```python
from build123d import *

# Parameters (mm, degrees)
BOSS_EXTRUDE1_DEPTH = 70
CHAMFER1_SIZE       = 7
FILLET1_R           = 2
SKETCH2_R           = 1.75
SKETCH2_R_2         = 20
CUT_EXTRUDE1_DEPTH  = 23
CUT_EXTRUDE2_START  = -4
SKETCH3_R           = 4.75
SKETCH3_R_2         = 1.75
CUT_EXTRUDE2_DEPTH  = 4
SKETCH5_R           = 20
CUT_EXTRUDE3_DEPTH  = 23


with BuildPart() as part:
    # Sketch1 → Boss-Extrude1 (new body)
    with BuildSketch(Plane.XY):
        Polygon((-55, 0), (0, 0), (0, 55), (-8, 55), (-8, 63), (8, 63), (8, -8), (-63, -8), (-63, 8), (-55, 8), align=None)
    extrude(amount=BOSS_EXTRUDE1_DEPTH)

    # Chamfer1
    chamfer1_edges = [part.edges().sort_by_distance(p)[0] for p in [
        (-8, 63, 35),
        (-63, 8, 35),
    ]]
    chamfer(chamfer1_edges, length=CHAMFER1_SIZE)

    # Fillet1
    fillet1_edges = [part.edges().sort_by_distance(p)[0] for p in [
        (8, 63, 35),
        (8, -8, 35),
        (-63, -8, 35),
    ]]
    fillet(fillet1_edges, radius=FILLET1_R)

    # Sketch2 → Cut-Extrude1 (cut)
    with BuildSketch(Plane.XZ.offset(8)):
        with Locations(Location((-40, 62.5, 0), (0, 0, 270))):
            Circle(SKETCH2_R)
        with Locations(Location((-15, 62.5, 0), (0, 0, 270))):
            Circle(SKETCH2_R)
        with Locations(Location((-15, 7.5, 0), (0, 0, 270))):
            Circle(SKETCH2_R)
        with Locations(Location((-40, 7.5, 0), (0, 0, 270))):
            Circle(SKETCH2_R)
        with Locations(Location((-27.5, 35, 0), (0, 0, 270))):
            Circle(SKETCH2_R_2)
    extrude(amount=-CUT_EXTRUDE1_DEPTH, mode=Mode.SUBTRACT)

    # Sketch3 → Cut-Extrude2 (cut)
    # profile 1 of 4: a face of its own
    with BuildSketch(Plane(origin=(0, 0, 0), x_dir=(1, 0, 0), z_dir=(0, 1, 0)).offset(CUT_EXTRUDE2_START)):
        with Locations(Location((-40, -62.5, 0), (0, 0, 270))):
            Circle(SKETCH3_R)
        with Locations(Location((-40, -62.5, 0), (0, 0, 90))):
            Circle(SKETCH3_R_2, mode=Mode.SUBTRACT)
    # profile 2 of 4: a face of its own
    with BuildSketch(Plane(origin=(0, 0, 0), x_dir=(1, 0, 0), z_dir=(0, 1, 0)).offset(CUT_EXTRUDE2_START)):
        with Locations(Location((-15, -62.5, 0), (0, 0, 270))):
            Circle(SKETCH3_R)
        with Locations(Location((-15, -62.5, 0), (0, 0, 90))):
            Circle(SKETCH3_R_2, mode=Mode.SUBTRACT)
    # profile 3 of 4: a face of its own
    with BuildSketch(Plane(origin=(0, 0, 0), x_dir=(1, 0, 0), z_dir=(0, 1, 0)).offset(CUT_EXTRUDE2_START)):
        with Locations(Location((-15, -7.5, 0), (0, 0, 270))):
            Circle(SKETCH3_R)
        with Locations(Location((-15, -7.5, 0), (0, 0, 90))):
            Circle(SKETCH3_R_2, mode=Mode.SUBTRACT)
    # profile 4 of 4: a face of its own
    with BuildSketch(Plane(origin=(0, 0, 0), x_dir=(1, 0, 0), z_dir=(0, 1, 0)).offset(CUT_EXTRUDE2_START)):
        with Locations(Location((-40, -7.5, 0), (0, 0, 270))):
            Circle(SKETCH3_R)
        with Locations(Location((-40, -7.5, 0), (0, 0, 90))):
            Circle(SKETCH3_R_2, mode=Mode.SUBTRACT)
    extrude(amount=CUT_EXTRUDE2_DEPTH, mode=Mode.SUBTRACT)

    # Sketch5 → Cut-Extrude3 (cut)
    with BuildSketch(Plane(origin=(8, 0, 0), x_dir=(0, 0, -1), z_dir=(1, 0, 0))):
        with Locations((-35, 27.5)):
            Circle(SKETCH5_R)
    extrude(amount=-CUT_EXTRUDE3_DEPTH, mode=Mode.SUBTRACT)


solid = part.part
```
Input: part model. Units: mm. Frame: model coordinates. A direction names the side the tool comes from. Give positions to 0.01 mm unless a question says otherwise; leave off trailing zeros. Order: outer loops, then holes, each group sorted by start corner. A loop starts at its lowest first (then second) coordinate and runs counter-clockwise, first axis right, second up. Notation, with made-up numbers: (74, -22.75) - (83, -22.75) arc R6 ccw to (83, -17.75) - close; hole circle Ø5 at (29.5, -2.75). An arc over 180 degrees is marked (long way). Use a Markdown table: item, result.
(1) Pin query (flat end, axial travel): pin 1 (1.5 mm diameter, centred on y = 3, z = 55, fed in from -X); pin 2 (0.5 mm diameter, centred on x = -55.5, z = 29.5, fed in from +Y); pin 3 (6 mm diameter, centred on x = -18.5, z = 17, fed in from +Y); pin 4 (3 mm diameter, centred on x = -40, z = 7.5, fed in from -Y). Return the tip coordinate at first contact, or that it passes through.
Computed values:
| item | result |
|---|---|
| pin 1 | stops at x = -61.75 |
| pin 2 | stops at y = 8 |
| pin 3 | stops at y = 0 |
| pin 4 | passes through |
(2) Draft query along Y for faces 1 (the cylindrical face through (4.056, 33.507, 15.924)), 2 (the cylindrical face through (-13.5, -6, 6.6)), 3 (the flat face through (-42, -4, 62)). Return one class per face: released by +Y, released by -Y, zero draft, split by the parting line, or undercut.
Computed values:
| item | result |
|---|---|
| face 1 | undercut |
| face 2 | zero draft |
| face 3 | released by +Y |
(3) Section query A-A (x = -4.5). Output: boundary loops of the cut face in (y, z).
Computed values:
| item | result |
|---|---|
| outline | (-8, 0) - (0, 0) - (0, 70) - (-8, 70) - close; (55, 0) - (59.5, 0) - (59.5, 70) - (55, 70) - close |
(4) Section query D-D (x = -15). Output: boundary loops of the cut face in (y, z), then the cut area to 3 significant figures.
Computed values:
| item | result |
|---|---|
| outline | (-8, 0) - (0, 0) - (0, 2.75) - (-4, 2.75) - (-4, 5.75) - (-8, 5.75) - close; (-8, 9.25) - (-4, 9.25) - (-4, 12.25) - (0, 12.25) - (0, 19.39) - (-8, 19.39) - close; (-8, 50.61) - (0, 50.61) - (0, 57.75) - (-4, 57.75) - (-4, 60.75) - (-8, 60.75) - close; (-8, 64.25) - (-4, 64.25) - (-4, 67.25) - (0, 67.25) - (0, 70) - (-8, 70) - close |
| area | 206 mm2 |
(5) Section query B-B (z = 23). Output: boundary loops of the cut face in (x, y), then the cut area to 3 significant figures.
Computed values:
| item | result |
|---|---|
| outline | (-63, -6) arc R2 ccw to (-61, -8) - (-43.5, -8) - (-43.5, 0) - (-55, 0) - (-55, 8) - (-56, 8) - (-63, 1) - close; (-11.5, -8) - (6, -8) arc R2 ccw to (8, -6) - (8, 11.5) - (0, 11.5) - (0, 0) - (-11.5, 0) - close; (-8, 55) - (0, 55) - (0, 43.5) - (8, 43.5) - (8, 61) arc R2 ccw to (6, 63) - (-1, 63) - (-8, 56) - close |
| area | 636 mm2 |
(6) Access query for faces 4 (the cylindrical face through (7.4, 62.43, 35.49)), 5 (the flat face through (-46, 0, 27)), 6 (the flat face through (-55, 4, 35)), 7 (the cylindrical face through (-14.791, -2.028, 2.755)). Directions: +Z, -Z, +X, -X, +Y, -Y. A direction counts if a zero-diameter tool reaches every point of the face in a straight line with its end or side. Return the directions, or none.
Computed values:
| item | result |
|---|---|
| face 4 | +Z, -Z, +X, +Y |
| face 5 | +Z, -Z |
| face 6 | +Z, -Z, +Y |
| face 7 | +Y |
(7) Line query: line 1 (X direction, y = -1.5, z = 62.5); line 2 (X direction, y = -6, z = 62); line 3 (X direction, y = -6, z = 35). Output: solid intervals per line, ascending. Write a range as from..to.
Computed values:
| item | result |
|---|---|
| line 1 | x = -63..-44.75, -35.25..-19.75, -10.25..8 |
| line 2 | x = -63..-41.68, -38.32..-16.68, -13.32..8 |
| line 3 | x = -63..-47.5, -7.5..8 |
(8) Section query C-C (y = 39.5). Output: boundary loops of the cut face in (x, z), then the cut area to 3 significant figures.
Computed values:
| item | result |
|---|---|
| outline | (0, 0) - (8, 0) - (8, 19) - (0, 19) - close; (0, 51) - (8, 51) - (8, 70) - (0, 70) - close |
| area | 304 mm2 |
